from build123d import *

# Parameters (mm, degrees)
F0_W      = 120
F0_H      = 85
F0_R      = 5.209452
F0_R_2    = 4.712977
F1_DEPTH  = 3
F2_W      = 120
F2_H      = 3
F3_DEPTH  = 52.5
F5_W      = 16.148806
F5_H      = 12.583495
F5_R      = 3.062628
F6_DEPTH  = 5
F7_R      = 5.08
F9_R      = 9.525
F10_DEPTH = 152.4
F11_W     = 2.430552
F11_H     = 84.969267
F12_DEPTH = 52.5
F13_R     = 12.7
F14_DEPTH = 25.4
F15_R     = 3.81
F16_DEPTH = 152.4


with BuildPart() as f1:
    # F0 (on Front) → F1 (new body)
    with BuildSketch(Plane.XZ):
        Rectangle(F0_W, F0_H)
        with Locations((-38.1, -14.170533)):
            Circle(F0_R, mode=Mode.SUBTRACT)
        with Locations((-12.7, -14.170533)):
            Circle(F0_R_2, mode=Mode.SUBTRACT)
        with Locations((12.7, -14.170533)):
            Circle(F0_R_2, mode=Mode.SUBTRACT)
        with Locations((38.1, -14.170533)):
            Circle(F0_R, mode=Mode.SUBTRACT)
        with Locations((-38.1, 14.170533)):
            Circle(F0_R, mode=Mode.SUBTRACT)
        with Locations((-12.7, 14.170533)):
            Circle(F0_R_2, mode=Mode.SUBTRACT)
        with Locations((12.7, 14.170533)):
            Circle(F0_R_2, mode=Mode.SUBTRACT)
        with Locations((38.1, 14.170533)):
            Circle(F0_R, mode=Mode.SUBTRACT)
    extrude(amount=F1_DEPTH)

    # F2 (on face) → F3 (join)
    with BuildSketch(Plane.XZ.offset(3)):
        with Locations((0, 41)):
            Rectangle(F2_W, F2_H)
    extrude(amount=F3_DEPTH)

    # F4: F1 across plane


with BuildPart() as f1_1:
    add(f1.part)
    add(f1.part.mirror(Plane.XY))

    # F5 (on face) → F6 (join)
    with BuildSketch(Plane.XZ.offset(55.5)):
        with Locations((0, 48.026971)):
            Rectangle(F5_W, F5_H)
        with Locations((0, 48.026972)):
            Circle(F5_R, mode=Mode.SUBTRACT)
    extrude(amount=-F6_DEPTH)

    # F7
    f7_edges = [f1_1.edges().sort_by_distance(p)[0] for p in [
        (-8.074403, -53, 42.5),
        (8.074403, -53, 42.5),
    ]]
    fillet(f7_edges, radius=F7_R)

    # F8: F1 across plane


with BuildPart() as f1_2:
    add(f1_1.part)
    add(f1_1.part.mirror(Plane.XY))

    # F9 (on face) → F10 (cut)
    with BuildSketch(Plane.XY.offset(42.5)):
        with Locations((-38.1, -27.75)):
            Circle(F9_R)
        with Locations((-12.7, -27.75)):
            Circle(F9_R)
        with Locations((12.7, -27.75)):
            Circle(F9_R)
        with Locations((38.1, -27.75)):
            Circle(F9_R)
    extrude(amount=-F10_DEPTH, mode=Mode.SUBTRACT)

    # F11 (on face) → F12 (join, through all)
    with BuildSketch(Plane.XZ.offset(3)):
        with Locations((-58.784724, -0.015367)):
            Rectangle(F11_W, F11_H)
    extrude(amount=F12_DEPTH)

    # F13 (on face) → F14 (cut)
    with BuildSketch(Plane(origin=(-60, 0, 0), x_dir=(0, -1, 0), z_dir=(-1, 0, 0))):
        with Locations((24.957247, 22.86)):
            Circle(F13_R)
        with Locations((24.957247, -22.86)):
            Circle(F13_R)
    extrude(amount=-F14_DEPTH, mode=Mode.SUBTRACT)

    # F15 (on face) → F16 (cut)
    with BuildSketch(Plane(origin=(0, 0, -42.5), x_dir=(1, 0, 0), z_dir=(0, 0, -1))):
        with Locations((53.270094, 50.753396)):
            Circle(F15_R)
        with Locations((53.270094, 37.75046)):
            Circle(F15_R)
        with Locations((53.270094, 23.069726)):
            Circle(F15_R)
        with Locations((53.270094, 9.018165)):
            Circle(F15_R)
    extrude(amount=-F16_DEPTH, mode=Mode.SUBTRACT)


solid = f1_2.part
Here's how the part is built. I have some questions about the finished solid (model axes, mm). A direction names the side the tool comes from. Coordinates: 2 decimals unless noted, no trailing zeros. Order: outer loops, then holes, each group sorted by start corner. A loop starts at its lowest first (then second) coordinate and runs counter-clockwise, first axis right, second up.
Item 1: If we section it at D-D on z = 26.5: List the corners of the cut face in (x, y) for me.
Result sheet:
outline: (-60, -55.5) - (-57.57, -55.5) - (-57.57, -37.12) - (-60, -37.12) - close; (-60, -12.79) - (-57.57, -12.79) - (-57.57, -3) - (60, -3) - (60, 0) - (-60, 0) - close
Item 2: For P1, Ø22, axis at x = 12.7, y = -27.75, coming from the -Z side; P2, Ø3, axis at x = 25, y = -35.5, coming from the +Z side; P3, Ø4, axis at y = -52, z = 52.5, coming from the -X side, each with a flat end and sliding along its axis, tell me the tip position at first contact or that it passes through.
Result sheet:
P1: stops at z = -42.5
P2: stops at z = 42.5
P3: stops at x = -8.07
Item 3: If we section it at B-B on y = -43.5: List the corners of the cut face in (x, z) for me.
Result sheet:
outline: (-60, -42.5) - (60, -42.5) - (60, -39.5) - (-57.57, -39.5) - (-57.57, 39.5) - (60, 39.5) - (60, 42.5) - (-60, 42.5) - close
Item 4: I need wall thicknesses on line 1 (Z direction, x = -38.1, y = -2.25); line 2 (Z direction, x = 0, y = -53.6); line 3 (Z direction, x = -10, y = -5.5). Which ranges of each line are inside material? Lowest first, please.
Result sheet:
line 1: z = -42.5 to -19.38, -8.96 to 8.96, 19.38 to 42.5
line 2: z = -54.32 to -51.09, -44.96 to -39.5, 39.5 to 44.96, 51.09 to 54.32
line 3: z = -42.5 to -39.5, 39.5 to 42.5
Item 5: If we mould it in two halves opening along X, with no side actions, what happens to faces 4 (the face through (9.52, -52.96, 44.03)), 5 (the face through (-17.41, -1.48, -13.96)), 6 (the face through (-58.802, -22.204, 10.462))? For each: +X half, -X half, draft (parallel to the pull), parting line (faces both ways), or undercut.
Result sheet:
face 4: +X half
face 5: undercut
face 6: draft
Item 6: If we section it at C-C on x = 0: List the corners of the cut face in (y, z) for me, plus the area to 3 significant figures.
Result sheet:
outline: (-55.5, -54.32) - (-50.5, -54.32) - (-50.5, -51.09) - (-55.5, -51.09) - close; (-55.5, -44.96) - (-50.5, -44.96) - (-50.5, -42.5) - (0, -42.5) - (0, 42.5) - (-50.5, 42.5) - (-50.5, 44.96) - (-55.5, 44.96) - (-55.5, 39.5) - (-3, 39.5) - (-3, -39.5) - (-55.5, -39.5) - close; (-55.5, 51.09) - (-50.5, 51.09) - (-50.5, 54.32) - (-55.5, 54.32) - close
area: 627 mm2
Item 7: For faces 1 (the face through (-57.569, -29, -1)), 2 (the face through (8.074, -53, -51)), 3 (the face through (56.904, -24.214, -41.021)), which set-ups out of +Z, -Z, +X, -X, +Y, -Y let a thin tool reach every point of the face, with its end or its side?
Result sheet:
face 1: +X, -Y
face 2: -Z, +X, +Y, -Y
face 3: +Z, -Z
Item 8: If we section it at A-A on x = 38.1: List the corners of the cut face in (y, z) for me (3 decimals).
Result sheet:
outline: (-55.5, -42.5) - (-37.275, -42.5) - (-37.275, -39.5) - (-55.5, -39.5) - close; (-55.5, 39.5) - (-37.275, 39.5) - (-37.275, 42.5) - (-55.5, 42.5) - close; (-18.225, -42.5) - (0, -42.5) - (0, -19.38) - (-3, -19.38) - (-3, -39.5) - (-18.225, -39.5) - close; (-18.225, 39.5) - (-3, 39.5) - (-3, 19.38) - (0, 19.38) - (0, 42.5) - (-18.225, 42.5) - close; (-3, -8.961) - (0, -8.961) - (0, 8.961) - (-3, 8.961) - close
